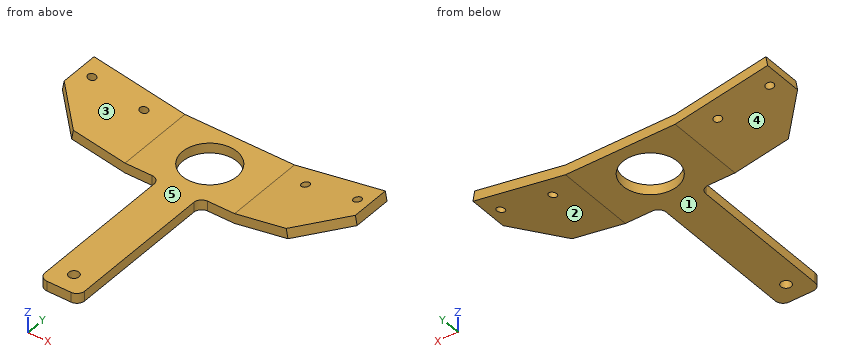
from build123d import *

# Parameters (mm, degrees)
SKETCH1_R           = 17.4
SKETCH1_R_2         = 3.265
BOSS_EXTRUDE1_DEPTH = 6.35
FILLET2_R           = 5
BOSS_EXTRUDE2_DEPTH = 50.8
CUT_EXTRUDE4_DEPTH  = 181.692673495
SKETCH8_R           = 2.575
CUT_EXTRUDE6_DEPTH  = 10


with BuildPart() as part:
    # Sketch1 → Boss-Extrude1 (new body)
    with BuildSketch(Plane.XY):
        Polygon((-12.7, 0), (12.7, 0), (12.7, 102.57), (35, 102.57), (35, 153.37), (-35, 153.37), (-35, 102.57), (-12.7, 102.57), align=None)
        with Locations((0, 127.97)):
            Circle(SKETCH1_R, mode=Mode.SUBTRACT)
        with Locations((0, 12.7)):
            Circle(SKETCH1_R_2, mode=Mode.SUBTRACT)
    extrude(amount=BOSS_EXTRUDE1_DEPTH)

    # Fillet2
    fillet2_edges = [part.edges().sort_by_distance(p)[0] for p in [
        (12.7, 102.57, 3.175),
        (12.7, 0, 3.175),
        (-12.7, 0, 3.175),
        (-12.7, 102.57, 3.175),
    ]]
    fillet(fillet2_edges, radius=FILLET2_R)

    # Sketch2 → Boss-Extrude2 (add)
    with BuildSketch(Plane(origin=(0, 153.37, 0), x_dir=(1, 0, 0), z_dir=(0, 1, 0))):
        Polygon((-35, 0), (-94.088465181, -10.41889066), (-93.002551226, -16.577414731), (-35, -6.35), align=None)
    boss_extrude2 = extrude(amount=-BOSS_EXTRUDE2_DEPTH)

    # Sketch6 → Cut-Extrude4 (cut, symmetric)
    with BuildSketch(Plane(origin=(0.030534819, 0, 0.173171563), x_dir=(0.9848077530122079, 0, -0.17364817766693147), z_dir=(0.17364817766693147, 0, 0.9848077530122079))):
        Polygon((-94.468271355, 102.57), (-94.468271355, 127.97), (-69.068271355, 102.57), align=None)
    cut_extrude4 = extrude(amount=CUT_EXTRUDE4_DEPTH, both=True, mode=Mode.SUBTRACT)

    # Mirror1: Boss-Extrude2, Cut-Extrude4 across plane
    add(boss_extrude2.mirror(Plane(origin=(0, 0, 0), x_dir=(0, 0, 1), z_dir=(1, 0, 0))))
    add(cut_extrude4.mirror(Plane(origin=(0, 0, 0), x_dir=(0, 0, 1), z_dir=(1, 0, 0))), mode=Mode.SUBTRACT)

    # Sketch8 → Cut-Extrude6 (cut)
    with BuildSketch(Plane(origin=(1.055379136, 0, -5.985352508), x_dir=(-0.9848077530122079, 0, -0.17364817766693139), z_dir=(0.17364817766693139, 0, -0.9848077530122079))):
        with Locations((-86.162231322, 140.67)):
            Circle(SKETCH8_R)
        with Locations((-52.434701963, 140.67)):
            Circle(SKETCH8_R)
    cut_extrude6 = extrude(amount=-CUT_EXTRUDE6_DEPTH, mode=Mode.SUBTRACT)

    # Mirror2: Cut-Extrude6 across plane
    add(cut_extrude6.mirror(Plane(origin=(0, 0, 0), x_dir=(0, 0, 1), z_dir=(1, 0, 0))), mode=Mode.SUBTRACT)


solid = part.part
Model file for the job. Use its own axes, mm. Face numbers are marked on the shaded views. A direction names the side the tool comes from. Give positions to 0.01 mm unless a question says otherwise; leave off trailing zeros. Write each loop counter-clockwise with the first axis right and the second up, starting at its lowest first coordinate (ties: lowest second). Pieces come first, ordered by that corner, then holes. Notation, with made-up numbers: M 38.5,7 L 53.5,7 A14 ccw 53.5,30 Z; hole C 42.5,32.5 d8. An arc over 180 degrees is marked long. One line per item, written item: value. Start each with the question number.
Q1. Saw through at A-A, the plane y = 12.7. Write the cut outline in (x, z) (3 decimals).
Q2. Two-plate mould, pull along X, no slides. Class the marked faces 1, 2 and 3: +X half, -X half, draft (parallel to the pull), parting line (faces both ways), or undercut.
Q3. 3-axis set-ups, long thin cutter, end or side, ignore diameter. For the marked faces 4 and 5: which of +Z, -Z, +X, -X, +Y, -Y reach the whole face in a straight line?
Q4. Saw through at D-D, the plane x = 73.5. Write the cut outline in (y, z).
Q5. Saw through at B-B, the plane x = 0. Write the cut outline in (y, z) (3 decimals).
Q6. Saw through at C-C, the plane y = 36. Write the cut outline in (x, z), plus the area to 3 significant figures.
Q7. Drop flat-ended pins along their axis: pin 1 Ø6 at (y, z) = (39.5, 5) entering from -X; pin 2 Ø6 at (y, z) = (137.5, 11) entering from +X; pin 3 Ø5 at (x, z) = (27.5, 5) entering from -Y. Give the stop position or say it passes through.
Q8. Probe probe 1 along Y at (x, z) = (0, 3) (3 decimals); probe 2 along X at (y, z) = (65.5, 1.75); probe 3 along Z at (x, y) = (30, 124). List the from-to ranges inside material, lowest first. Write a range as [from, to].
Output values:
1. outline: M -12.7,0 L -3.265,0 L -3.265,6.35 L -12.7,6.35 Z; M 3.265,0 L 12.7,0 L 12.7,6.35 L 3.265,6.35 Z
2. face 1: draft
2. face 2: +X half
2. face 3: undercut
3. face 4: -Z, -X, +Y, -Y
3. face 5: +Z, +Y, -Y
4. outline: M 107.06,6.79 L 153.37,6.79 L 153.37,13.14 L 108.17,13.14 Z
5. outline: M 0,0 L 9.435,0 L 9.435,6.35 L 0,6.35 Z; M 15.965,0 L 110.57,0 L 110.57,6.35 L 15.965,6.35 Z; M 145.37,0 L 153.37,0 L 153.37,6.35 L 145.37,6.35 Z
6. outline: M -12.7,0 L 12.7,0 L 12.7,6.35 L -12.7,6.35 Z
6. area: 161 mm²
7. pin 1: stops at x = -12.7
7. pin 2: stops at x = 94.09
7. pin 3: stops at y = 102.57
8. probe 1: y = [0, 9.435], [15.965, 110.57], [145.37, 153.37]
8. probe 2: x = [-12.7, 12.7]
8. probe 3: z = [0, 6.35]
